Autodesk Inventor part; units mm, degrees
ref_plane "YZ Plane" through (0, 0, 0) normal (1, 0, 0) x (0, 1, 0)
ref_plane "XZ Plane" through (0, 0, 0) normal (0, 1, 0) x (-1, 0, 0)
ref_plane "XY Plane" through (0, 0, 0) normal (0, 0, 1) x (1, 0, 0)
sketch "Sketch1" plane through (0, 0, 0) normal (0, 1, 0) x (-1, 0, 0)
  line L0 (-50, -122.5) -> (50, -122.5)
  line L1 (50, -122.5) -> (50, -47.5)
  line L2 (50, -47.5) -> (-50, -47.5)
  line L3 (-50, -47.5) -> (-50, -122.5)
  line L4 (-50, -122.5) -> (50, -47.5) construction
  line L5 (50, -122.5) -> (-50, -47.5) construction
  line L6 (-325, 122.5) -> (-225, 122.5)
  line L7 (-225, 122.5) -> (-225, 47.5)
  line L8 (-225, 47.5) -> (-325, 47.5)
  line L9 (-325, 47.5) -> (-325, 122.5)
  line L10 (-325, 122.5) -> (-225, 47.5) construction
  line L11 (-225, 122.5) -> (-325, 47.5) construction
  line L12 (0, 214.4175) -> (0, -235.835)
  line L13 (325, 122.5) -> (225, 122.5)
  line L14 (225, 122.5) -> (225, 47.5)
  line L15 (225, 47.5) -> (325, 47.5)
  line L16 (325, 47.5) -> (325, 122.5)
  line L17 (325, 122.5) -> (225, 47.5) construction
  line L18 (225, 122.5) -> (325, 47.5) construction
  point P0 (0, 0)
  point P1 (0, -85)
  point P2 (-275, 85)
  point P3 (275, 85)
  dimension "d0" = 100
  dimension "d1" = 75
  dimension "d2" = 85
  dimension "d3" = 100
  dimension "d4" = 75
  dimension "d5" = 275
  dimension "d6" = 85
sketch "Sketch2" plane through (0, 0, 0) normal (0, 1, 0) x (-1, 0, 0)
  line L0 (-7.5, -95) -> (7.5, -95)
  line L1 (7.5, -95) -> (7.5, -75)
  line L2 (7.5, -75) -> (-7.5, -75)
  line L3 (-7.5, -75) -> (-7.5, -95)
  line L4 (267.5, 95) -> (267.5, 75)
  line L5 (267.5, 75) -> (282.5, 75)
  line L6 (282.5, 75) -> (282.5, 95)
  line L7 (282.5, 95) -> (267.5, 95)
  line L8 (-267.5, 95) -> (-282.5, 95)
  line L9 (-282.5, 95) -> (-282.5, 75)
  line L10 (-282.5, 75) -> (-267.5, 75)
  line L11 (-267.5, 75) -> (-267.5, 95)
  line L12 (-137.5, -150) -> (137.5, -150)
  line L13 (137.5, -150) -> (137.5, -200)
  line L14 (137.5, -200) -> (-137.5, -200)
  line L15 (-137.5, -200) -> (-137.5, -150)
  line L16 (-137.5, -150) -> (137.5, -200) construction
  line L17 (137.5, -150) -> (-137.5, -200) construction
  arc A0 (-376.4677, -20.0539) -> (-137.5, -150) centre (-137.5, 134.7009) ccw
  line L18 (-137.5, -150) -> (-137.5, 134.7009) construction
  line L19 (-412.5, 61.0149) -> (-137.5, 134.7009) construction
  arc A1 (-412.5, -56.0862) -> (-137.5, -200) centre (-137.5, 134.7009) ccw
  line L20 (0, -269.3547) -> (0, -73.2831)
  arc A2 (137.5, -150) -> (376.4677, -20.0539) centre (137.5, 134.7009) ccw
  arc A3 (137.5, -200) -> (412.5, -56.0862) centre (137.5, 134.7009) ccw
  line L21 (412.5, -56.0862) -> (376.4677, -20.0539)
  line L22 (412.5, -56.0862) -> (463.4573, -56.0862) construction
  line L23 (-412.5, -56.0862) -> (-376.4677, -20.0539)
  point P0 (0, 0)
  point P1 (0, -175)
  point P2 (412.5, 61.0149)
  dimension "d9" = 275
  dimension "d10" = 50
  dimension "d11" = 100
  dimension "d12" = 75
  dimension "d17" = 135
extrude "Extrusion2" add sketch "Sketch2" along normal blind 100 contours L12 L13 L14 L20 | L20 L14 L15 L12 | L15 A1 L23 A0 | A2 L21 A3 L13
fillet "Fillet1" radius 3 12 edges at (0, 100, -150) (273.507, 100, -115.4125) (-273.507, 100, -115.4125) (-394.4839, 100, -38.07) (394.4839, 100, -38.07) (-376.4677, 50, -20.0539) (-412.5, 50, -56.0862) (376.4677, 50, -20.0539) (412.5, 50, -56.0862) (-292.6904, 100, -161.847) (292.6904, 100, -161.847) (0, 100, -200)
sketch "Sketch3" plane through (0, 0, 0) normal (0, -1, 0) x (1, 0, 0)
  line L0 (350, 188.4615) -> (-350, 188.4615)
  line L1 (-350, 188.4615) -> (-350, -54.7677)
  line L2 (350, -54.7677) -> (350, 188.4615)
  arc A0 (411.0516, -58.1571) -> (410.721, -54.3072) centre (408.5997, -56.4285) ccw
  line L3 (379.0735, -22.6597) -> (410.721, -54.3072)
  arc A1 (379.0735, -22.6597) -> (374.4553, -23.118) centre (376.9522, -24.781) ccw
  arc A2 (137.5, -150) -> (374.4553, -23.118) centre (137.5, 134.7009) ccw
  line L4 (-137.5, -150) -> (137.5, -150)
  arc A3 (-374.4553, -23.118) -> (-137.5, -150) centre (-137.5, 134.7009) ccw
  arc A4 (-374.4553, -23.118) -> (-379.0735, -22.6597) centre (-376.9522, -24.781) ccw
  line L5 (-410.721, -54.3072) -> (-379.0735, -22.6597)
  arc A5 (-410.721, -54.3072) -> (-411.0516, -58.1571) centre (-408.5997, -56.4285) ccw
  arc A6 (-411.0516, -58.1571) -> (-137.5, -200) centre (-137.5, 134.7009) ccw
  line L6 (137.5, -200) -> (-137.5, -200)
  arc A7 (137.5, -200) -> (411.0516, -58.1571) centre (137.5, 134.7009) ccw
  arc A8 (137.5, -200) -> (411.0516, -58.1571) centre (137.5, 134.7009) ccw
  line L7 (0, -256.7037) -> (0, -18.0297)
  point P0 (0, 0)
  dimension "d31" = 700
extrude "Extrusion3" add sketch "Sketch3" against normal blind 2 contours L2 A2 L4 A3 L1 L0
extrude "Extrusion6" add sketch "Sketch1" along normal blind 20
sketch "Sketch6" plane through (325, 2, 47.5) normal (1, 0, 0) x (0, 0, -1)
  line L0 (0, 0) -> (-75, 0)
  line L1 (0, 0) -> (0, 18)
  line L2 (-75, 18) -> (0, 18)
  line L3 (-75, 0) -> (-75, 18)
  line L4 (0, 0) -> (0, 18)
  line L5 (0, 18) -> (-75, 9)
  line L6 (-75, 0) -> (-75, 18)
  line L7 (-75, 18) -> (0, 18)
  line L8 (-75, 9) -> (-75, 18)
  point P0 (47.5, -2)
extrude "Extrusion7" cut sketch "Sketch6" against normal through all contours L5 L3 L2
sketch "Sketch7" plane through (50, 2, -122.5) normal (1, 0, 0) x (0, 0, -1)
  line L0 (0, 0) -> (-75, 0)
  line L1 (0, 0) -> (0, 18)
  line L2 (-75, 18) -> (0, 18)
  line L3 (-75, 0) -> (-75, 18)
  line L4 (0, 18) -> (-75, 9)
  line L5 (-75, 9) -> (-75, 18)
  line L6 (-75, 18) -> (0, 18)
  line L7 (-75, 18) -> (0, 18)
  point P0 (-122.5, -2)
extrude "Extrusion8" cut sketch "Sketch7" against normal up to surface (100 mm away) contours L4 L3 L2
properties part number "Charging Dock" material "ABS Plastic"
Geometry: final body of the model. Coordinates: model frame, mm. A direction names the side the tool comes from. Give positions to 0.01 mm unless a question says otherwise; leave off trailing zeros. Loops run counter-clockwise (first coordinate to the right, second up) from the corner with the lowest first, then second, coordinate; pieces in that order, holes last. Notation, with made-up numbers: (23.25, -15) -> (76.25, -15) arc R24 ccw to (76.25, 10) -> close; hole circle Ø3 at (18.5, 13.5). An arc over 180 degrees is marked (long way). Put each result on its own line as item: value.
1. Cut plane C-C (z = -1). Return the cut outline in (x, y).
Taken from the geometry:
outline: (-350, 0) -> (350, 0) -> (350, 2) -> (-350, 2) -> close
2. Cut plane A-A (x = 88). Return the cut outline in (y, z), plus the area to 3 significant figures.
Taken from the geometry:
outline: (0, -200) -> (97, -200) arc R3 ccw to (100, -197) -> (100, -153) arc R3 ccw to (97, -150) -> (2, -150) -> (2, 188.46) -> (0, 188.46) -> close
area: 5,670 mm2
3. Ray query, line 1 along Y through (x, z) = (77, -4); line 2 along X through (y, z) = (14, -117); line 3 along X through (y, z) = (39, -100.5). Return the intervals inside material, ascending. Write a range as [from, to].
Taken from the geometry:
line 1: y = [0, 2]
line 2: x = [-358.12, -270.55], [-50, 50], [270.55, 358.12]
line 3: x = [-375.63, -297.92], [297.92, 375.63]
4. Cut plane B-B (y = 33). Return the cut outline in (x, z), plus the area to 3 significant figures.
Taken from the geometry:
outline: (-411.05, -58.16) arc R334.7 ccw to (-137.5, -200) -> (137.5, -200) arc R334.7 ccw to (411.05, -58.16) arc R3 ccw to (410.72, -54.31) -> (379.07, -22.66) arc R3 ccw to (374.46, -23.12) arc R284.7 cw to (137.5, -150) -> (-137.5, -150) arc R284.7 cw to (-374.46, -23.12) arc R3 ccw to (-379.07, -22.66) -> (-410.72, -54.31) arc R3 ccw to start
area: 44,100 mm2
5. Pin query (flat end, axial travel): P1, Ø9, axis at y = 11.5, z = 89.5, coming from the -X side; P2, Ø20, axis at y = 12, z = -91.5, coming from the +X side; P3, Ø6, axis at x = 275.5, y = 20, coming from the -Z side; P4, Ø12, axis at x = 249.5, z = -152.5, coming from the -Y side. Return the tip coordinate at first contact, or that it passes through.
Taken from the geometry:
P1: stops at x = -325
P2: stops at x = 393
P3: stops at z = -171.57
P4: stops at y = 0
6. Set-up query: faces 1 (the flat face through (-274.3, 15.563, 84.475)), 2 (the flat face through (274, 11, 47.5)), 3 (the flat face through (-325, 9, 84)), 4 (the flat face through (1, 11, -122.5)), 5 (the flat face through (-225, 9, 86)). Return all of +Z, -Z, +X, -X, +Y, -Y with unobstructed straight access to the full face (end or side cutting, diameter ignored); none if empty.
Taken from the geometry:
face 1: +Z, +X, -X, +Y
face 2: +X, -X, +Y
face 3: +Z, -X, +Y
face 4: +Y
face 5: +Z, +Y
